Design review of the part shown in the three views and the two pictorial views. Dimensions are in mm from the part's minimum x, y and z. A direction names the side the tool comes from. Coordinates: 2 decimals unless noted, no trailing zeros. Order: outer loops, then holes, each group sorted by start corner. A loop starts at its lowest first (then second) coordinate and runs counter-clockwise, first axis right, second up. Notation, with made-up numbers: (55, 6) -> (107, 6) arc R18 cw to (107, 39) -> close; hole circle Ø2 at (-28.5, -1.5). An arc over 180 degrees is marked (long way). Answer as CSV lines item,"result". Start each with the question number.
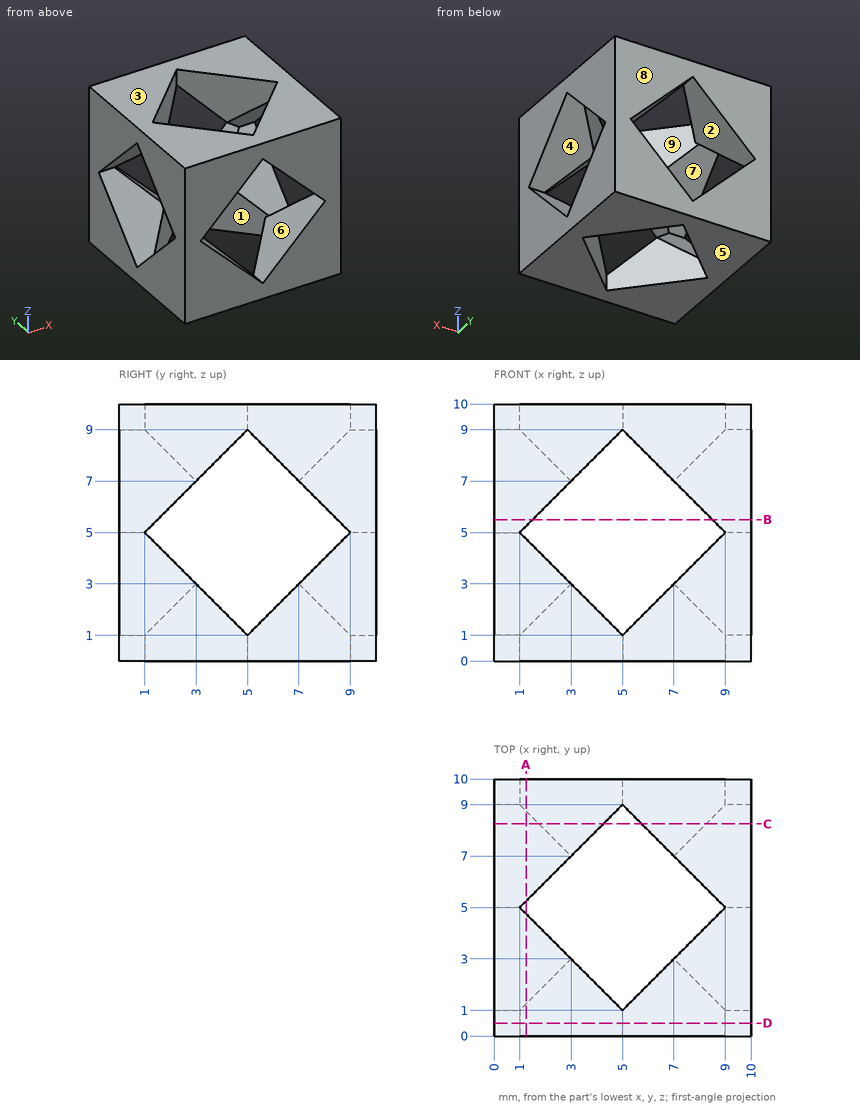
1) Consider section C-C (y = 8.25). Give the boundary of the cut face in (x, z), plus the area to 4 significant figures.
2) Tool access review of the marked faces 5, 6, 7, 8 and 9: name each direction out of +Z, -Z, +X, -X, +Y, -Y from which nothing blocks a thin tool from reaching the whole face with its end or side.
3) Consider section A-A (x = 1.25). Give the boundary of the cut face in (y, z).
4) Wall thickness on L1, parallel to Z at x = 7, y = 1.75; L2, parallel to Z at x = 1.5, y = 2: over which ranges is each line inside the solid? List them lowest first. Write a range as [from, to].
5) Consider section B-B (z = 5.5). Give the boundary of the cut face in (x, y).
6) Mouldability with a two-part tool opening along Z and no side actions: class the marked faces 1, 2, 3 and 4 as released by +Z, released by -Z, zero draft, split by the parting line, or undercut.
7) Consider section D-D (y = 0.5). Give the boundary of the cut face in (x, z).
Result:
1,outline,"(0, 0) -> (4.25, 0) -> (4.25, 1.75) -> (1.75, 4.25) -> (0, 4.25) -> close; (0, 5.75) -> (1.75, 5.75) -> (4.25, 8.25) -> (4.25, 10) -> (0, 10) -> close; (5.75, 0) -> (10, 0) -> (10, 4.25) -> (8.25, 4.25) -> (5.75, 1.75) -> close; (5.75, 8.25) -> (8.25, 5.75) -> (10, 5.75) -> (10, 10) -> (5.75, 10) -> close"
1,area,"59.75 mm2"
2,face 5,"-Z, +X, -X, +Y, -Y"
2,face 6,"+Y, -Y"
2,face 7,"+X, -X"
2,face 8,"+Z, -Z, +X, -X, +Y"
2,face 9,"+Z, -Z"
3,outline,"(0, 0) -> (4.75, 0) -> (4.75, 1.25) -> (1.25, 4.75) -> (0, 4.75) -> close; (0, 5.25) -> (1.25, 5.25) -> (4.75, 8.75) -> (4.75, 10) -> (0, 10) -> close; (5.25, 0) -> (10, 0) -> (10, 4.75) -> (8.75, 4.75) -> (5.25, 1.25) -> close; (5.25, 8.75) -> (8.75, 5.25) -> (10, 5.25) -> (10, 10) -> (5.25, 10) -> close"
4,L1,"[0, 3], [7, 10]"
4,L2,"[0, 4], [6, 10]"
5,outline,"(0, 0) -> (1.5, 0) -> (1.5, 1.5) -> (0, 1.5) -> close; (0, 8.5) -> (1.5, 8.5) -> (1.5, 10) -> (0, 10) -> close; (8.5, 0) -> (10, 0) -> (10, 1.5) -> (8.5, 1.5) -> close; (8.5, 8.5) -> (10, 8.5) -> (10, 10) -> (8.5, 10) -> close"
6,face 1,"zero draft"
6,face 2,"undercut"
6,face 3,"released by +Z"
6,face 4,"undercut"
7,outline,"(0, 0) -> (10, 0) -> (10, 10) -> (0, 10) -> close; hole (1, 5) -> (5, 1) -> (9, 5) -> (5, 9) -> close"
